Source: three-view drawing plus pictorial views. Frame: mm from the lowest corner of the part. Coordinates: 2 decimals unless noted, no trailing zeros. Order: outer loops, then holes, each group sorted by start corner. A loop starts at its lowest first (then second) coordinate and runs counter-clockwise, first axis right, second up. Notation, with made-up numbers: (87, 72.25) - (104, 72.25) arc R22 ccw to (104, 88.25) - close; hole circle Ø5 at (-14.5, -19). An arc over 180 degrees is marked (long way). One line per question, with ' | ' between items.
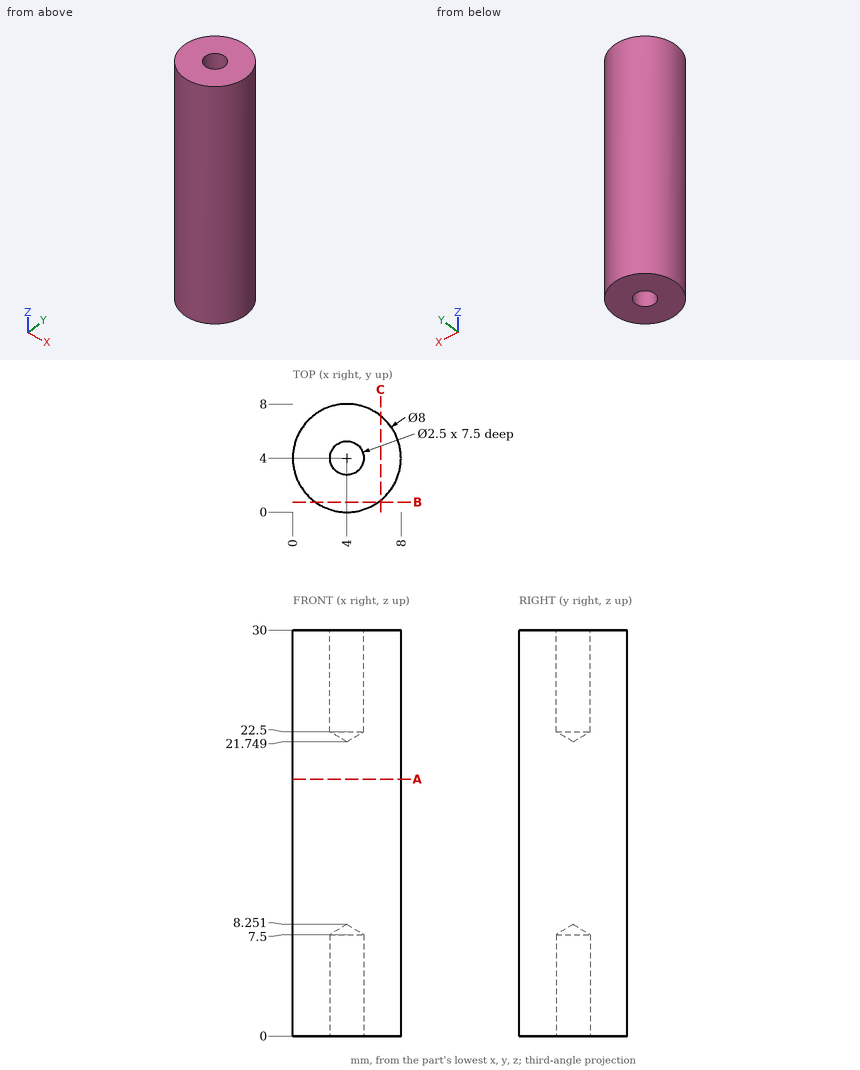
Item 1: Ray query, line 1 (X direction, y = 4.75, z = 4.25); line 2 (Y direction, x = 3, z = 25); line 3 (Y direction, x = 1, z = 17.5). Return the intervals inside material, ascending.
Data:
line 1: 0.07 to 3, 5 to 7.93 | line 2: 0.13 to 3.25, 4.75 to 7.87 | line 3: 1.35 to 6.65
Item 2: Section A-A on z = 19. Return the cut outline in (x, y), and give its area (3 significant figures).
Data:
outline: circle Ø8 at (4, 4) | area: 50.3 mm^2
Item 3: Contact query for flat-ended pins moving along their axis: P1, Ø3, axis at y = 1, z = 6, coming from the -X side; P2, Ø1, axis at y = 7, z = 21.5, coming from the -X side; P3, Ø2, axis at x = 4, y = 4, coming from the -Z side. Output: stop coordinate, or through.
Data:
P1: x = 0.29 | P2: x = 0.88 | P3: z = 7.65
Item 4: Section B-B on y = 0.75. Return the cut outline in (x, z), and give its area (3 significant figures).
Data:
outline: (1.67, 0) - (6.33, 0) - (6.33, 30) - (1.67, 30) - close | area: 140 mm^2
Item 5: Section C-C on x = 6.5. Return the cut outline in (y, z).
Data:
outline: (0.88, 0) - (7.12, 0) - (7.12, 30) - (0.88, 30) - close
